Build history of the part. All positions in model axes, mm. Face numbers are marked on the shaded views. A direction names the side the tool comes from. Round coordinates to 2 decimals unless told otherwise and drop trailing zeros. Write each loop counter-clockwise with the first axis right and the second up, starting at its lowest first coordinate (ties: lowest second). Pieces come first, ordered by that corner, then holes.
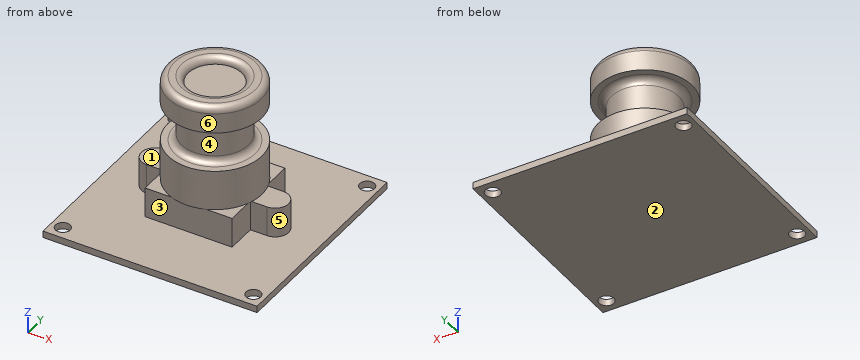
from build123d import *

# Parameters (mm, degrees)
SKETCH_2_W          = 32
SKETCH_2_H          = 32
SKETCH_2_R          = 1.1
EXTRUDE_1_DEPTH     = 1
EXTRUDE_2_DEPTH     = 4.5
SKETCH_4_R          = 7
EXTRUDE_3_DEPTH     = 6
SKETCH_5_R          = 5
EXTRUDE_4_DEPTH     = 6
SKETCH_6_R          = 7
EXTRUDE_5_DEPTH     = 4
SKETCH_9_R          = 4
CUT_EXTRUDE_2_DEPTH = 1
FILLET_2_R          = 1


with BuildPart() as part:
    # 草图2 → 凸台-拉伸1 (new body)
    with BuildSketch(Plane.XY):
        Rectangle(SKETCH_2_W, SKETCH_2_H)
        with Locations((-14.25, -14)):
            Circle(SKETCH_2_R, mode=Mode.SUBTRACT)
        with Locations((-14.25, 14)):
            Circle(SKETCH_2_R, mode=Mode.SUBTRACT)
        with Locations(Location((14.25, 14, 0), (0, 0, 180))):
            Circle(SKETCH_2_R, mode=Mode.SUBTRACT)
        with Locations(Location((14.25, -14, 0), (0, 0, 180))):
            Circle(SKETCH_2_R, mode=Mode.SUBTRACT)
    extrude(amount=EXTRUDE_1_DEPTH)

    # 草图3 → 凸台-拉伸2 (add)
    with BuildSketch(Plane.XY.offset(1)):
        with BuildLine():
            Line((-6.5, -6.5), (6.5, -6.5))
            Line((6.5, -6.5), (6.5, -2))
            Line((6.5, -2), (9, -2))
            ThreePointArc((9, -2), (11, 0), (9, 2))
            Line((9, 2), (6.5, 2))
            Line((6.5, 2), (6.5, 6.5))
            Line((6.5, 6.5), (-6.5, 6.5))
            Line((-6.5, 6.5), (-6.5, 2))
            Line((-6.5, 2), (-9, 2))
            ThreePointArc((-9, 2), (-11, 0), (-9, -2))
            Line((-9, -2), (-6.5, -2))
            Line((-6.5, -2), (-6.5, -6.5))
        make_face()
    extrude(amount=EXTRUDE_2_DEPTH)

    # 草图4 → 凸台-拉伸3 (add)
    with BuildSketch(Plane.XY.offset(5.5)):
        with Locations(Location((0, 0, 0), (0, 0, 196.601549599))):
            Circle(SKETCH_4_R)
    extrude(amount=EXTRUDE_3_DEPTH)

    # 草图5 → 凸台-拉伸4 (add)
    with BuildSketch(Plane.XY.offset(11.5)):
        Circle(SKETCH_5_R)
    extrude(amount=EXTRUDE_4_DEPTH)

    # 草图6 → 凸台-拉伸5 (add)
    with BuildSketch(Plane.XY.offset(17.5)):
        with Locations(Location((0, 0, 0), (0, 0, 196.601549599))):
            Circle(SKETCH_6_R)
    extrude(amount=EXTRUDE_5_DEPTH)

    # 草图9 → 切除-拉伸2 (cut)
    with BuildSketch(Plane.XY.offset(21.5)):
        Circle(SKETCH_9_R)
    extrude(amount=-CUT_EXTRUDE_2_DEPTH, mode=Mode.SUBTRACT)

    # 圆角2
    fillet_2_edges = [part.edges().sort_by_distance(p)[0] for p in [
        (-4, 0, 21.5),
        (-5, 0, 11.5),
        (-5, 0, 17.5),
        (6.708203933, 2, 21.5),
    ]]
    fillet(fillet_2_edges, radius=FILLET_2_R - 0.0001)  # a hair under: the kernel refuses the full size


solid = part.part
1) Pin check, flat tips, straight feed: pin 1 Ø2 at (x, y) = (8.5, 0) entering from +Z; pin 2 Ø4 at (x, z) = (9.5, 4.5) entering from +Y; pin 3 Ø8 at (x, z) = (-8, 9.5) entering from +Y; pin 4 Ø3 at (x, y) = (5, 4.5) entering from +Z. Stop position of each tip, or through.
Results:
pin 1: stops at z = 5.5
pin 2: stops at y = 2
pin 3: stops at y = 5.74
pin 4: stops at z = 21.5
2) Mould opens along Z. For the marked faces 1, 2 and 3 say: released by +Z, released by -Z, zero draft, split by the parting line, or undercut.
Results:
face 1: released by +Z
face 2: released by -Z
face 3: undercut
3) Slice it at C-C (z = 2.75). Write the cut outline in (x, y).
Results:
outline: (-9, -2) - (-6.5, -2) - (-6.5, -6.5) - (6.5, -6.5) - (6.5, -2) - (9, -2) arc R2 ccw to (9, 2) - (6.5, 2) - (6.5, 6.5) - (-6.5, 6.5) - (-6.5, 2) - (-9, 2) arc R2 ccw to start
4) Which spindle directions (+Z, -Z, +X, -X, +Y, -Y) get a long thin tool onto all of the face, cutting with end or side? Do the marked faces 4, 5 and 6. Say none if no direction does.
Results:
face 4: none
face 5: +Z, +X
face 6: +Z
5) Slice it at A-A (y = 14). Write the cut outline in (x, z), plus the area to 3 significant figures.
Results:
outline: (-16, 0) - (-15.35, 0) - (-15.35, 1) - (-16, 1) - close; (-13.15, 0) - (13.15, 0) - (13.15, 1) - (-13.15, 1) - close; (15.35, 0) - (16, 0) - (16, 1) - (15.35, 1) - close
area: 27.6 mm2
6) Wall check: L1, parallel to Y at x = -14.25, z = 0.8; L2, parallel to Z at x = 6.5, y = 14.5; L3, parallel to Y at x = 8.5, z = 3.75. Give the ranges that are in metal, low to high.
Results:
L1: y = -16 to -15.1, -12.9 to 12.9, 15.1 to 16
L2: z = 0 to 1
L3: y = -2 to 2
7) Slice it at D-D (x = 14). Write the cut outline in (y, z).
Results:
outline: (-16, 0) - (-15.07, 0) - (-15.07, 1) - (-16, 1) - close; (-12.93, 0) - (12.93, 0) - (12.93, 1) - (-12.93, 1) - close; (15.07, 0) - (16, 0) - (16, 1) - (15.07, 1) - close
